Could you check a few things on this model? Use its own coordinates, in mm. A direction names the side the tool comes from. Coordinates: 2 decimals unless noted, no trailing zeros. Write each loop counter-clockwise with the first axis right and the second up, starting at its lowest first coordinate (ties: lowest second). Pieces come first, ordered by that corner, then holes. Notation, with made-up numbers: (85, 6) - (142, 6) arc R18 ccw to (142, 22) - close; hole circle Ø9 at (79.25, 14). An arc over 180 degrees is marked (long way). Answer as a JSON object with one key per item and string values. Group by question number.
1) Will these pins go through, and if not, where does the flat tip stop? pin 1 Ø12.5 at (x, z) = (-1.5, 42.5) entering from +Y; pin 2 Ø1.5 at (x, z) = (5.5, 29) entering from -Y; pin 3 Ø1.5 at (y, z) = (1, 29) entering from +X.
2) If we section it at A-A (x = 13.5): Write out the boundary of the cut face in (y, z), plus the area to 3 significant figures.
3) If we section it at D-D (x = -9): Write out the boundary of the cut face in (y, z).
4) Please list where these lines run through material, in increasing order: line 1 along X through (y, z) = (17, 48.5); line 2 along Z through (x, y) = (22.5, 9); line 3 along Y through (x, z) = (-22, 39.5).
5) If we section it at B-B (z = 22.5): Write out the boundary of the cut face in (x, y), plus the area to 3 significant figures.
6) On a 3-axis mill with a long thin cutter (end or side, diameter ignored), from which of +Z, -Z, +X, -X, +Y, -Y can I reach the whole of each face in a straight line? I mean faces 1 (the flat face through (0, -6, 28)), 2 (the flat face through (-21, 10, 36)), 3 (the flat face through (0, 6, 28)). Say none if no direction works.
Autodesk Fusion 360 part; units mm, degrees
sketch "Sketch1" plane through (0, 0, 0) normal (0, 0, 1) x (1, 0, 0)
  line L0 (-33, -21) -> (33, -21)
  line L1 (33, -21) -> (33, 21)
  line L2 (33, 21) -> (-33, 21)
  line L3 (-33, 21) -> (-33, -21)
  line L4 (-33, -21) -> (33, 21) construction
  line L5 (33, -21) -> (-33, 21) construction
  dimension "d1" = 66
  dimension "d2" = 42
extrude "Extrude1" add sketch "Sketch1" along normal blind 12
chamfer "Chamfer1" distance 12 angle 45 2 edges at (33, -21, 6) (33, 21, 6)
sketch "Sketch2" plane through (0, 0, 12) normal (0, 0, 1) x (-1, 0, 0)
  line L0 (-33, -9) -> (-21, -21)
  line L1 (-21, -21) -> (33, -21)
  line L2 (33, -21) -> (33, 21)
  line L3 (33, 21) -> (-21, 21)
  line L4 (-21, 21) -> (-33, 9)
  line L5 (-33, 9) -> (-33, -9)
  line L6 (33, -21) -> (21, -21)
  line L7 (21, -21) -> (21, 21)
  line L8 (21, 21) -> (33, 21)
  line L9 (33, 21) -> (33, -21)
  dimension "d6" = 12
extrude "Extrude2" add sketch "Sketch2" along normal blind 48 contours L1 L2 L3 L6 L7 L8 L9
fillet "Fillet1" radius 21 2 edges at (-27, -21, 60) (-27, 21, 60)
sketch "Sketch3" plane through (0, 0, 0) normal (0, 1, 0) x (1, 0, 0)
  line L0 (-21.1163, -54.0232) -> (-21.1163, -12.0232)
  line L1 (-21.1163, -12.0232) -> (32.8837, -12.0232)
  line L2 (32.8837, -12.0232) -> (-21.1163, -54.0232)
  dimension "d11" = 42
  dimension "d12" = 54
extrude "Extrude3" add sketch "Sketch3" along normal mid plane 12
Here are the results:
{
 "1": {"pin 1": "stops at y = 6", "pin 2": "stops at y = -6", "pin 3": "stops at x = 12.02"},
 "2": {"outline": "(-21, 0) - (21, 0) - (21, 12) - (-21, 12) - close; (-6, 12.02) - (6, 12.02) - (6, 27.1) - (-6, 27.1) - close", "area": "685 mm²"},
 "3": {"outline": "(-21, 0) - (21, 0) - (21, 12) - (-21, 12) - close; (-6, 12.02) - (6, 12.02) - (6, 44.6) - (-6, 44.6) - close"},
 "4": {"line 1": "x = -33 to -21", "line 2": "z = 0 to 12", "line 3": "y = -20.99 to 20.99"},
 "5": {"outline": "(-33, -21) - (-21, -21) - (-21, -6) - (19.41, -6) - (19.41, 6) - (-21, 6) - (-21, 21) - (-33, 21) - close", "area": "989 mm²"},
 "6": {"face 1": "+Z, +X, -Y", "face 2": "+Z, +X", "face 3": "+Z, +X, +Y"}
}
